```python
from build123d import *

# Parameters (mm, degrees)
SKETCH3_W           = 14.2
SKETCH3_H           = 14.2
BOSS_EXTRUDE1_DEPTH = 4.5


with BuildPart() as part:
    # Sketch2 → Revolve1 (revolve)
    with BuildSketch(Plane.XY):
        with BuildLine():
            Line((0, 0), (0, 13))
            ThreePointArc((0, 13), (3.296209945, 12.350752265), (6.1, 10.5))
            Line((6.1, 10.5), (7.1, 10.5))
            Line((7.1, 10.5), (7.1, 8))
            Line((7.1, 8), (5.1, 8))
            Line((5.1, 8), (5.1, 5.5))
            Line((5.1, 5.5), (7.1, 5.5))
            Line((7.1, 5.5), (7.1, 0))
            Line((7.1, 0), (0, 0))
        make_face()
    revolve(axis=Axis((0, 0, 0), (0, 1, 0)))

    # Sketch3 → Boss-Extrude1 (add)
    with BuildSketch(Plane(origin=(0, 0, 0), x_dir=(1, 0, 0), z_dir=(0, 1, 0))):
        Rectangle(SKETCH3_W, SKETCH3_H)
    extrude(amount=-BOSS_EXTRUDE1_DEPTH)


solid = part.part
```
Geometry check sheet. Reference: the model listing, model coordinates, mm. A direction names the side the tool comes from. Coordinates: 2 decimals unless noted, no trailing zeros. Write each loop counter-clockwise with the first axis right and the second up, starting at its lowest first coordinate (ties: lowest second). Pieces come first, ordered by that corner, then holes. Notation, with made-up numbers: M -2.75,12 L 16.25,12 A23 ccw 16.25,42 Z; hole C -35,36.5 d10. An arc over 180 degrees is marked long. One line per item, written item: value. Start each with the question number.
(1) Release check for a two-part mould opening along Y. For faces 4 (the face through (-0.92, 9.23, -7.04)), 5 (the face through (6, 0, 6)), 6 (the face through (5, 5.5, -2)) record: released by +Y, released by -Y, zero draft, split by the parting line, or undercut.
(2) Sectioned sample at B-B, the plane z = 3.5. Enter the section's corners in (x, y).
(3) Sectioned sample at C-C, the plane x = -1.25. Enter the section's corners in (y, z), and give its area (3 significant figures).
(4) Scan lines: line 1 along Y through (x, z) = (-3.75, 5.5); line 2 along Y through (x, z) = (1.5, 1.5); line 3 along Y through (x, z) = (1.25, -4.5). Record each from-to range of solid material in increasing order. Write a range as [from, to].
(5) Tool access check on faces 1 (the face through (-6, 0, 5)), 2 (the face through (-2, 10.5, -6)), 3 (the face through (2.4, 6.7, 4.5)). Record the directions out of +Z, -Z, +X, -X, +Y, -Y that give a thin tool (end or side, any length) a straight path to the whole face; none if there is none.
(6) Sectioned sample at D-D, the plane y = 2.75. Enter the section's corners in (x, z).
(7) Sectioned sample at A-A, the plane x = -5.5. Enter the section's corners in (y, z).
(8) Depth check by flat-ended pin: pin 1 (8 mm diameter, centred on x = -5, z = 4.5, fed in from +Y); pin 2 (8 mm diameter, centred on x = 4.5, z = -2, fed in from +Y); pin 3 (1.5 mm diameter, centred on y = 5.5, z = 2, fed in from -X). Enter the tip coordinate at first touch or a pass-through.
Filled sheet:
1. face 4: zero draft
1. face 5: released by +Y
1. face 6: undercut
2. outline: M -7.1,-4.5 L 7.1,-4.5 L 7.1,0 L 6.18,0 L 6.18,5.5 L 3.71,5.5 L 3.71,8 L 6.18,8 L 6.18,10.5 L 5,10.5 A7.96 ccw -5,10.5 L -6.18,10.5 L -6.18,8 L -3.71,8 L -3.71,5.5 L -6.18,5.5 L -6.18,0 L -7.1,0 Z
3. outline: M -4.5,-7.1 L 0,-7.1 L 0,-6.99 L 5.5,-6.99 L 5.5,-4.94 L 8,-4.94 L 8,-6.99 L 10.5,-6.99 L 10.5,-5.97 A8.6 ccw 10.5,5.97 L 10.5,6.99 L 8,6.99 L 8,4.94 L 5.5,4.94 L 5.5,6.99 L 0,6.99 L 0,7.1 L -4.5,7.1 Z
3. area: 220 mm²
4. line 1: [-4.5, 5.5], [8, 10.5]
4. line 2: [-4.5, 12.74]
4. line 3: [-4.5, 11.64]
5. face 1: +Z, -X, +Y
5. face 2: +Y
5. face 3: none
6. outline: C 0,0 d14.2
7. outline: M -4.5,-7.1 L 0,-7.1 L 0,-4.49 L 5.5,-4.49 L 5.5,4.49 L 0,4.49 L 0,7.1 L -4.5,7.1 Z; M 8,-4.49 L 10.5,-4.49 L 10.5,-2.64 A6.73 ccw 10.5,2.64 L 10.5,4.49 L 8,4.49 Z
8. pin 1: y = 12.56
8. pin 2: y = 12.95
8. pin 3: x = -6.99
